Source: CAD feature listing. Evaluate the final solid. Frame: model axes, mm. A direction names the side the tool comes from. Round coordinates to 2 decimals unless told otherwise and drop trailing zeros. Loops run counter-clockwise (first coordinate to the right, second up) from the corner with the lowest first, then second, coordinate; pieces in that order, holes last. Notation, with made-up numbers: (-21, 15) -> (-10, 15) arc R28 ccw to (-10, 47) -> close; hole circle Ø1 at (-7, -10.75). An arc over 180 degrees is marked (long way). Put each result on its own line as item: value. Start each with the question number.
1. Draft query along Z for faces 1 (the cylindrical face through (-0.58, -0.54, 2.44)), 2 (the flat face through (-1.06, 0, 0)), 3 (the flat face through (0, 2, 1)). Return one class per face: pulls with the +Z half, pulls with the -Z half, needs draft (parallel to the pull), parting line crosses it, or undercut.
2. Cut plane A-A (x = 5.75). Return the cut outline in (y, z).
3. Contact query for flat-ended pins moving along their axis: pin 1 (1 mm diameter, centred on y = -1.5, z = -1, fed in from -X); pin 2 (0.6 mm diameter, centred on y = -0.5, z = 0, fed in from -X); pin 3 (1 mm diameter, centred on x = 7.5, z = -0.5, fed in from +Y). Output: stop coordinate, or through.
4. Material intervals for L1, parallel to Z at x = 8.75, y = -0.05; L2, parallel to X at y = 0.05, z = 0.6, sorted ascending.
5. Set-up query: faces 4 (the flat face through (10, 0, 0)), 5 (the cylindrical face through (5.51, -0.27, -1.22)). Return all of +Z, -Z, +X, -X, +Y, -Y with unobstructed straight access to the full face (end or side cutting, diameter ignored); none if empty.
Autodesk Inventor part; units mm, degrees
ref_plane "YZ Plane" through (0, 0, 0) normal (1, 0, 0) x (0, 1, 0)
ref_plane "XZ Plane" through (0, 0, 0) normal (0, 1, 0) x (-1, 0, 0)
ref_plane "XY Plane" through (0, 0, 0) normal (0, 0, 1) x (1, 0, 0)
sketch "Sketch4" plane through (0, 0, 0) normal (0, 0, 1) x (1, 0, 0)
  line L0 (-2.1, 0) -> (10, 0)
  line L1 (0, 0) -> (-2.1, 0)
  line L2 (0, 2.5) -> (0, 1.725)
  line L3 (0.5, 1.225) -> (0.5, 1.225)
  line L4 (0.5, 1.225) -> (0.9, 1.25)
  arc A0 (0, 1.725) -> (0.5, 1.225) centre (0.5, 1.725) ccw
  line L5 (-2.1, 0) -> (-2.1, 1.25)
  line L6 (0, 2.5) -> (-1.1375, 2.5)
  arc A1 (-1.1375, 2.5) -> (-2.1, 1.25) centre (1.4883, -0.5175) ccw
  line L7 (0.9, 1.25) -> (10, 1.25)
  line L8 (10, 1.25) -> (10, 0)
  point P0 (0, 1.225)
  dimension "d71" = 0.5
  dimension "d72" = 10
  dimension "d74" = 0.4
  dimension "d75" = 2.45
  dimension "d78" = 2.5
  dimension "d82" = 4
  dimension "d83" = 2.1
  dimension "d84" = 5
  dimension "d104" = 9.1
  dimension "d105" = 2.5
revolve "Revolution7" add sketch "Sketch4" angle 360 about axis through (-2.1, 0, 0) along (1, 0, 0)
sketch "Sketch5" plane through (-2.1, 0, 0) normal (-1, 0, 0) x (0, 0, 1)
  circle A0 centre (0, 0) radius 1.2 construction
  circle A1 centre (0, 0) radius 0.84 construction
  line L0 (0, 0) -> (-0.7275, 0.42)
  line L1 (0, 0) -> (-0.7275, -0.42)
  line L2 (-1.8008, 0) -> (1.7887, 0)
  line L3 (-1.2, 0) -> (-0.7275, -0.42)
  line L4 (-1.2, 0) -> (-0.7275, 0.42)
  dimension "d88" = 2.4
  dimension "d89" = 1.68
  dimension "d90" = 30
  dimension "d91" = 30
extrude "Extrusion1" cut sketch "Sketch5" against normal blind 1.04
pattern_circular "Circular Pattern1" count 6 over 360 about axis through (-10, 0, 0) along (1, 0, 0) of "Extrusion1"
fillet "Fillet1" radius 0.24 12 edges at (-1.58, -1.0392, -0.6) (-1.58, -0.42, -0.7275) (-1.58, -0.84, 0) (-1.58, -1.0392, 0.6) (-1.58, -0.42, 0.7275) (-1.58, 0, 1.2) (-1.58, 0.84, 0) (-1.58, 1.0392, 0.6) (-1.58, 0.42, 0.7275) (-1.58, 0.42, -0.7275) (-1.58, 0, -1.2) (-1.58, 1.0392, -0.6)
thread "Thread7"
properties part number "Flachkopfschraube mit Innenrund ISO 14583 - M2,5 x 10 - 4.8" material "Steel"
Solution:
1. face 1: parting line crosses it
1. face 2: undercut
1. face 3: needs draft
2. outline: circle Ø2.5 at (0, 0)
3. pin 1: stops at x = -2.07
3. pin 2: stops at x = -1.06
3. pin 3: stops at y = 1.25
4. L1: z = -1.25 to 1.25
4. L2: x = -1.06 to 10
5. face 4: +Z, -Z, +X, +Y, -Y
5. face 5: +X
